Check sheet for the drawn part. Datum: minimum x, y, z corner. Units: mm. A direction names the side the tool comes from. Round coordinates to 2 decimals unless told otherwise and drop trailing zeros. Write each loop counter-clockwise with the first axis right and the second up, starting at its lowest first coordinate (ties: lowest second). Pieces come first, ordered by that corner, then holes. Notation, with made-up numbers: (-38, 67.5) - (-7, 67.5) arc R19 ccw to (-7, 101.5) - close; hole circle Ø9 at (-32, 37.25). An arc over 180 degrees is marked (long way). Answer as a JSON object with one key per item and string values.
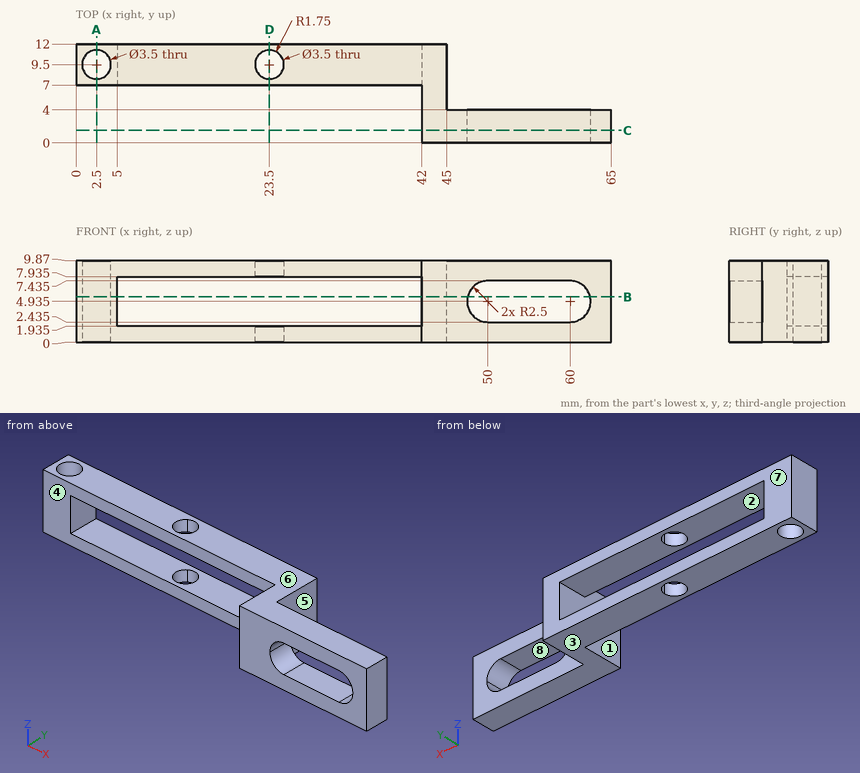
Q1. Set-up check for the marked faces 1, 2, 3, 4 and 5: record each of +Z, -Z, +X, -X, +Y, -Y from which the full face is reachable in a straight line by a thin tool's end or side.
Geometry check:
{"face 1": "-Y", "face 2": "+Y, -Y", "face 3": "-Z, +X, -X, +Y, -Y", "face 4": "+Z, -Z, -X, -Y", "face 5": "+Z, -Z, +X, +Y"}
Q2. Release check for a two-part mould opening along Z. For the marked faces 6, 7 and 8 record: released by +Z, released by -Z, zero draft, split by the parting line, or undercut.
Geometry check:
{"face 6": "released by +Z", "face 7": "zero draft", "face 8": "undercut"}
Q3. Section check A-A, the plane x = 2.5. Record the cut outline in (y, z).
Geometry check:
{"outline": "(7, 0) - (7.75, 0) - (7.75, 9.87) - (7, 9.87) - close; (11.25, 0) - (12, 0) - (12, 9.87) - (11.25, 9.87) - close"}
Q4. Gauge pin test, flat ends, axial feed: P1, Ø2.5, axis at y = 8.5, z = 3.5, coming from the +X side; P2, Ø3, axis at x = 23.5, y = 9.5, coming from the +Z side; P3, Ø5.5, axis at x = 22.5, y = 10, coming from the -Z side. Record the tip position at first contact, or that the pin passes through.
Geometry check:
{"P1": "stops at x = 45", "P2": "passes through", "P3": "stops at z = 0"}
Q5. Section check C-C, the plane y = 1.5. Record the cut outline in (x, z) (3 decimals).
Geometry check:
{"outline": "(42, 0) - (65, 0) - (65, 9.87) - (42, 9.87) - close; hole (50, 2.435) - (60, 2.435) arc R2.5 ccw to (60, 7.435) - (50, 7.435) arc R2.5 ccw to start"}
Q6. Section check D-D, the plane x = 23.5. Record the cut outline in (y, z) (3 decimals), then the cut area to 4 significant figures.
Geometry check:
{"outline": "(7, 0) - (7.75, 0) - (7.75, 1.935) - (7, 1.935) - close; (7, 7.935) - (7.75, 7.935) - (7.75, 9.87) - (7, 9.87) - close; (11.25, 0) - (12, 0) - (12, 1.935) - (11.25, 1.935) - close; (11.25, 7.935) - (12, 7.935) - (12, 9.87) - (11.25, 9.87) - close", "area": "5.805 mm2"}
Q7. Section check B-B, the plane z = 5.5. Record the cut outline in (x, y), then the cut area to 3 significant figures.
Geometry check:
{"outline": "(0, 7) - (5, 7) - (5, 12) - (0, 12) - close; (42, 0) - (47.56, 0) - (47.56, 4) - (45, 4) - (45, 12) - (42, 12) - close; (62.44, 0) - (65, 0) - (65, 4) - (62.44, 4) - close; hole circle Ø3.5 at (2.5, 9.5)", "area": "71.9 mm2"}
Q8. Material ranges on line 1 along X through (y, z) = (9.5, 4.25); line 2 along X through (y, z) = (9.5, 0.75); line 3 along Z through (x, y) = (32, 9.75) (3 decimals), recorded low to high. Write a range as [from, to].
Geometry check:
{"line 1": "x = [0, 0.75], [4.25, 5], [42, 45]", "line 2": "x = [0, 0.75], [4.25, 21.75], [25.25, 45]", "line 3": "z = [0, 1.935], [7.935, 9.87]"}
